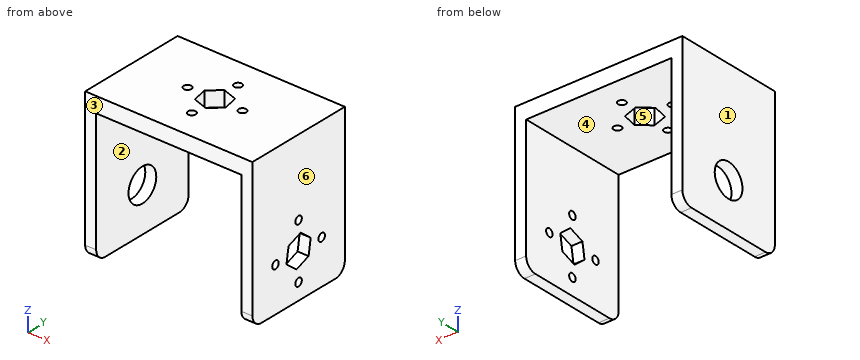
```python
from build123d import *

# Parameters (mm, degrees)
BOSS_EXTRUDE1_DEPTH = 50
SKETCH3_R           = 7.5
CUT_EXTRUDE1_DEPTH  = 5
CUT_EXTRUDE2_DEPTH  = 5
CUT_EXTRUDE3_DEPTH  = 7
SKETCH4_3_R         = 1.75
CUT_EXTRUDE4_DEPTH  = 5
SKETCH5_3_R         = 1.75
CUT_EXTRUDE6_DEPTH  = 7
FILLET1_R           = 5


with BuildPart() as part:
    # Sketch1 → Boss-Extrude1 (new body)
    with BuildSketch(Plane(origin=(0, 0, 0), x_dir=(1, 0, 0), z_dir=(0, 1, 0))):
        Polygon((0, 0), (33.03, 0), (33.03, 60), (38.03, 60), (38.03, -7), (-38.03, -7), (-38.03, 60), (-33.03, 60), (-33.03, 0), align=None)
    extrude(amount=BOSS_EXTRUDE1_DEPTH)

    # Sketch3 → Cut-Extrude1 (cut)
    with BuildSketch(Plane(origin=(-33.03, 0, 0), x_dir=(0, 0, -1), z_dir=(1, 0, 0))):
        with Locations((40, 25)):
            Circle(SKETCH3_R)
    extrude(amount=-CUT_EXTRUDE1_DEPTH, mode=Mode.SUBTRACT)

    # Sketch4 → Cut-Extrude2 (cut)
    with BuildSketch(Plane.ZY.offset(-33.03)):
        Polygon((-46.907161244, 23.863723826), (-42.46953659, 18.450084807), (-35.562375345, 19.586360981), (-33.092838756, 26.136276174), (-37.53046341, 31.549915193), (-44.437624655, 30.413639019), align=None)
    extrude(amount=-CUT_EXTRUDE2_DEPTH, mode=Mode.SUBTRACT)

    # Sketch5 → Cut-Extrude3 (cut)
    with BuildSketch(Plane(origin=(0, 0, 0), x_dir=(-1, 0, 0), z_dir=(0, 0, -1))):
        Polygon((1.451740182, 31.847806251), (-5.204504082, 29.681147002), (-6.656244264, 22.833340752), (-1.451740182, 18.152193749), (5.204504082, 20.318852998), (6.656244264, 27.166659248), align=None)
    extrude(amount=-CUT_EXTRUDE3_DEPTH, mode=Mode.SUBTRACT)

    # Sketch4<3> → Cut-Extrude4 (cut)
    with BuildSketch(Plane.ZY.offset(-33.03)):
        with Locations((-52.5, 25)):
            Circle(SKETCH4_3_R)
        with Locations((-40, 37.5)):
            Circle(SKETCH4_3_R)
        with Locations((-40, 12.5)):
            Circle(SKETCH4_3_R)
        with Locations((-27.5, 25)):
            Circle(SKETCH4_3_R)
    extrude(amount=-CUT_EXTRUDE4_DEPTH, mode=Mode.SUBTRACT)

    # Sketch5<3> → Cut-Extrude6 (cut)
    with BuildSketch(Plane(origin=(0, 0, 0), x_dir=(-1, 0, 0), z_dir=(0, 0, -1))):
        with Locations((0, 37.5)):
            Circle(SKETCH5_3_R)
        with Locations((-12.5, 25)):
            Circle(SKETCH5_3_R)
        with Locations((0, 12.5)):
            Circle(SKETCH5_3_R)
        with Locations((12.5, 25)):
            Circle(SKETCH5_3_R)
    extrude(amount=-CUT_EXTRUDE6_DEPTH, mode=Mode.SUBTRACT)

    # Fillet1
    fillet1_edges = [part.edges().sort_by_distance(p)[0] for p in [
        (35.53, 0, -60),
        (-35.53, 0, -60),
        (-35.53, 50, -60),
        (35.53, 50, -60),
    ]]
    fillet(fillet1_edges, radius=FILLET1_R)


solid = part.part
```
The listing builds one solid part. Answer for the finished solid, in the listing's coordinates (mm). Face numbers are marked on the shaded views. A direction names the side the tool comes from. Give positions to 0.01 mm unless a question says otherwise; leave off trailing zeros. Loops run counter-clockwise (first coordinate to the right, second up) from the corner with the lowest first, then second, coordinate; pieces in that order, holes last. Notation, with made-up numbers: M -2,60.5 L 29,60.5 A25 ccw 29,89.5 Z; hole C 33.25,-29 d9. An arc over 180 degrees is marked long. One line per item, written item: value.
1. Section C-C on x = -3 is taken. Determine the outline of the cut face in (y, z).
Found:
outline: M 0,0 L 19.6,0 L 19.6,7 L 0,7 Z; M 30.46,0 L 50,0 L 50,7 L 30.46,7 Z
2. Section A-A on y = 37.5 is taken. Determine the outline of the cut face in (x, z), plus the area to 3 significant figures.
Found:
outline: M -38.03,-60 L -33.03,-60 L -33.03,0 L -1.75,0 L -1.75,7 L -38.03,7 Z; M 1.75,0 L 33.03,0 L 33.03,-38.25 L 38.03,-38.25 L 38.03,7 L 1.75,7 Z; M 33.03,-60 L 38.03,-60 L 38.03,-41.75 L 33.03,-41.75 Z
area: 1,090 mm^2
3. Find the intervals of material crossed by probe 1 along Y at (x, z) = (34, -40); probe 2 along X at (y, z) = (35.5, -40); probe 3 along Y at (x, z) = (-12.5, 4.25), in increasing order.
Found:
probe 1: 0 to 10.75, 14.25 to 18.86, 31.14 to 35.75, 39.25 to 50
probe 2: -38.03 to -33.03, 33.03 to 38.03
probe 3: 0 to 23.25, 26.75 to 50
4. For the marked faces 4, 5 and 6, determine the directions among +Z, -Z, +X, -X, +Y, -Y from which every point of the face is accessible in a straight line to the end or side of a thin tool.
Found:
face 4: -Z, +Y, -Y
face 5: +Z, -Z
face 6: +Z, -Z, +X, +Y, -Y
5. Section B-B on z = -11 is taken. Determine the outline of the cut face in (x, y).
Found:
outline: M -38.03,0 L -33.03,0 L -33.03,50 L -38.03,50 Z; M 33.03,0 L 38.03,0 L 38.03,50 L 33.03,50 Z
6. Each of these flat-tipped pins is pushed along its axis until it touches: P1, Ø4, axis at x = 0, y = 12.5, coming from the +Z side; P2, Ø3, axis at y = 25, z = -52.5, coming from the +X side; P3, Ø4, axis at x = 6.5, y = 13.5, coming from the -Z side. Where does it stop, or does it pass through?
Found:
P1: z = 7
P2: x = -33.03
P3: z = 0
7. Section D-D on z = -27.5 is taken. Determine the outline of the cut face in (x, y), plus the area to 4 significant figures.
Found:
outline: M -38.03,0 L -33.03,0 L -33.03,50 L -38.03,50 Z; M 33.03,0 L 38.03,0 L 38.03,23.25 L 33.03,23.25 Z; M 33.03,26.75 L 38.03,26.75 L 38.03,50 L 33.03,50 Z
area: 482.5 mm^2
8. For a pull along X with two mould halves and no side action, classify the marked faces 1, 2 and 3 as pulls with the +X half, pulls with the -X half, needs draft (parallel to the pull), parting line crosses it, or undercut.
Found:
face 1: pulls with the -X half
face 2: undercut
face 3: needs draft
